The listing builds one solid part. Answer for the finished solid, in the listing's coordinates (mm). Face numbers are marked on the shaded views. Give positions to 0.01 mm unless a question says otherwise; leave off trailing zeros. Order: outer loops, then holes, each group sorted by start corner. A loop starts at its lowest first (then second) coordinate and runs counter-clockwise, first axis right, second up. Notation, with made-up numbers: (65.25, 49.5) - (94.25, 49.5) arc R22 cw to (94.25, 61.5) - close; hole circle Ø3 at (80.25, 53). An arc over 180 degrees is marked (long way). Answer as CSV lines item,"result". Start each with the question number.
1. Determine the mould class of the marked faces 1, 2 and 3 for opening direction Y: +Y half, -Y half, draft (parallel to the pull), parting line (faces both ways), or undercut.
2. Section A-A on z = 1.2 is taken. Give the vertices of the cut face in (x, y), and give its area (3 significant figures).
3. Flat-ended cylindrical pins translate along their axes: pin 1 (0.7 mm diameter, centred on x = 13.5, y = 11, fed in from -Z); pin 2 (2 mm diameter, centred on x = 1.5, y = -6.5, fed in from -Z). Find the tip coordinate at first contact, or state that the pin passes through.
4. Consider line 1 along X through (y, z) = (3.25, 1.45); line 2 along X through (y, z) = (-9, -1.1); line 3 along Z through (x, y) = (4, -7.75). Determine where each line is inside the solid, lowest interval first. Write a range as [from, to].
5. Section B-B on z = -0.55 is taken. Give the vertices of the cut face in (x, y), and give its area (3 significant figures).
Autodesk Inventor part; units mm, degrees
ref_plane "YZ Plane" through (0, 0, 0) normal (1, 0, 0) x (0, 1, 0)
ref_plane "XZ Plane" through (0, 0, 0) normal (0, 1, 0) x (-1, 0, 0)
ref_plane "XY Plane" through (0, 0, 0) normal (0, 0, 1) x (1, 0, 0)
ref_plane "Work Plane1" through (0, 0, 0) normal (0, 0, 1) x (1, 0, 0)
sketch "Sketch1" plane through (0, 0, 0) normal (0, 0, 1) x (1, 0, 0)
  circle A0 centre (11.8906, 0.2887) radius 14 construction
  line L0 (-4.1094, 7.6362) -> (-12.7094, 0.2473) construction
  line L1 (-5.7094, 0.2473) -> (-12.7094, 0.2473) construction
  line L2 (-5.7094, -6.0861) -> (-5.7094, 0.2473) construction
  line L3 (-6.0301, -6.0861) -> (-5.7094, -6.0861) construction
  line L4 (-6.0301, -6.0861) -> (-4.1094, -7.5697) construction
  line L5 (-4.1094, -7.5697) -> (-4.1094, -15.7113) construction
  line L6 (-4.1094, -15.7113) -> (27.8906, -15.7113) construction
  line L7 (27.8906, -15.7113) -> (27.8906, -7.5697) construction
  line L8 (29.8113, -6.0861) -> (27.8906, -7.5697) construction
  line L9 (29.4906, -6.0861) -> (29.8113, -6.0861) construction
  line L10 (29.4906, 0.2473) -> (29.4906, -6.0861) construction
  line L11 (36.4906, 0.2473) -> (29.4906, 0.2473) construction
  line L12 (27.8906, 7.6362) -> (36.4906, 0.2473) construction
  line L13 (27.8906, 7.6362) -> (27.8906, 16.2887) construction
  line L14 (27.8906, 16.2887) -> (-4.1094, 16.2887) construction
  line L15 (-4.1094, 16.2887) -> (-4.1094, 7.6362) construction
  circle A1 centre (11.8906, 0.2887) radius 13.9
  circle A2 centre (11.8906, 0.2887) radius 12.5
  point P0 (0, 0)
  dimension "d0" = 27.8
  dimension "d1" = 25
extrude "Extrusion1" add sketch "Sketch1" against normal blind 3 draft -2
sketch "Sketch2" plane through (11.8906, 0.2887, 0) normal (0, 0, 1) x (1, 0, 0)
  circle A0 centre (0, 0) radius 13.9
  circle A1 centre (0, 0) radius 12.5
  line L0 (17, -14) -> (-17, -14)
  line L1 (-17, -14) -> (-17, 14)
  line L2 (-17, 14) -> (17, 14)
  line L3 (17, 14) -> (17, -14)
  line L4 (17, -14) -> (-17, 14) construction
  line L5 (-17, -14) -> (17, 14) construction
  circle A2 centre (0, 0) radius 10.25 construction
  line L6 (-7.1545, 10.25) -> (7.1545, 10.25)
  line L7 (-12.454, 1.071) -> (-5.2995, -11.321)
  line L8 (5.2995, -11.321) -> (12.454, 1.071)
  point P0 (-11.8906, -0.2887)
  dimension "d4" = 34
  dimension "d5" = 28
  dimension "d8" = 20.5
  dimension "d9" = 60
  dimension "d10" = 60
  dimension "d11" = 0
extrude "Extrusion2" add sketch "Sketch2" along normal blind 2 contours A0 | A1 L8 | L6 A1 | A1 L7 | L0 L1 L2 L3
properties part number "20_Cube_Insert_Z-Focus_objectivemount"
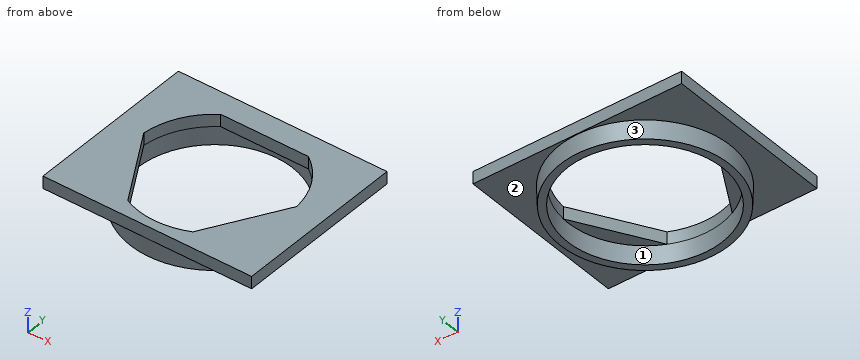
Checks:
1,face 1,"undercut"
1,face 2,"draft"
1,face 3,"parting line"
2,outline,"(-5.11, -13.71) - (28.89, -13.71) - (28.89, 14.29) - (-5.11, 14.29) - close; hole (-0.56, 1.36) - (6.59, -11.03) arc R12.5 ccw to (17.19, -11.03) - (24.34, 1.36) arc R12.5 ccw to (19.05, 10.54) - (4.74, 10.54) arc R12.5 ccw to start"
2,area,"527 mm²"
3,pin 1,"stops at z = 0"
3,pin 2,"stops at z = -3"
4,line 1,"x = [-5.11, -0.25], [24.03, 28.89]"
4,line 2,"x = [1.6, 3.47], [20.31, 22.18]"
4,line 3,"z = [0, 2]"
5,outline,"circle Ø27.76 at (11.89, 0.29); hole circle Ø25.04 at (11.89, 0.29)"
5,area,"113 mm²"
